```python
from build123d import *

# Parameters (mm, degrees)
SKETCH_1_W          = 26
SKETCH_1_H          = 38
EXTRUDE_1_DEPTH     = 12
SKETCH_2_W          = 22
SKETCH_2_H          = 34
CUT_EXTRUDE_1_DEPTH = 10
SKETCH_3_W          = 2
SKETCH_3_H          = 7
CUT_EXTRUDE_3_DEPTH = 12
SKETCH_4_W          = 6
SKETCH_4_H          = 6
EXTRUDE_2_DEPTH     = 5
SKETCH_5_R          = 1
CUT_EXTRUDE_4_DEPTH = 13
CUT_EXTRUDE_START   = 1
CUT_EXTRUDE_5_DEPTH = 4
SKETCH_7_R          = 12
SKETCH_7_R_2        = 11
EXTRUDE_3_DEPTH     = 5
SKETCH_9_W          = 8
SKETCH_9_H          = 15
CUT_EXTRUDE_7_DEPTH = 1
SKETCH_10_W         = 14.41096837
SKETCH_10_H         = 3
EXTRUDE_4_DEPTH     = 2


with BuildPart() as part:
    # ｽｹｯﾁ1 → ﾎﾞｽ - 押し出し1 (new body)
    with BuildSketch(Plane.XY):
        Rectangle(SKETCH_1_W, SKETCH_1_H)
    extrude(amount=EXTRUDE_1_DEPTH)

    # ｽｹｯﾁ2 → ｶｯﾄ - 押し出し1 (cut)
    with BuildSketch(Plane.XY):
        Rectangle(SKETCH_2_W, SKETCH_2_H)
    extrude(amount=CUT_EXTRUDE_1_DEPTH, mode=Mode.SUBTRACT)

    # ｽｹｯﾁ3 → ｶｯﾄ - 押し出し3 (cut)
    with BuildSketch(Plane.XY):
        with Locations((0.147807357, 5.5)):
            Rectangle(SKETCH_3_W, SKETCH_3_H)
    extrude(amount=CUT_EXTRUDE_3_DEPTH, mode=Mode.SUBTRACT)

    # ｽｹｯﾁ4 → ﾎﾞｽ - 押し出し2 (add)
    with BuildSketch(Plane.XY):
        with Locations((16, 16)):
            Rectangle(SKETCH_4_W, SKETCH_4_H)
        with Locations((16, -16)):
            Rectangle(SKETCH_4_W, SKETCH_4_H)
        with Locations((-16, -16)):
            Rectangle(SKETCH_4_W, SKETCH_4_H)
        with Locations((-16, 16)):
            Rectangle(SKETCH_4_W, SKETCH_4_H)
    extrude(amount=EXTRUDE_2_DEPTH)

    # ｽｹｯﾁ5 → ｶｯﾄ - 押し出し4 (cut, through all)
    with BuildSketch(Plane.XY):
        with Locations((-16, 16)):
            Circle(SKETCH_5_R)
        with Locations((-16, -16)):
            Circle(SKETCH_5_R)
        with Locations((16, -16)):
            Circle(SKETCH_5_R)
        with Locations((16, 16)):
            Circle(SKETCH_5_R)
    extrude(amount=CUT_EXTRUDE_4_DEPTH, mode=Mode.SUBTRACT)

    # ｽｹｯﾁ6 → ｶｯﾄ - 押し出し5 (cut)
    with BuildSketch(Plane.XY.offset(CUT_EXTRUDE_START)):
        Polygon((-17.184124892, 17.98272075), (-18.309148984, 15.965878137), (-17.125024092, 13.983157387), (-14.815875108, 14.01727925), (-13.690851016, 16.034121863), (-14.874975908, 18.016842613), align=None)
        Polygon((-17.07560545, -13.956374239), (-18.307634549, -15.909688764), (-17.2320291, -17.953314524), (-14.92439455, -18.043625761), (-13.692365451, -16.090311236), (-14.7679709, -14.046685476), align=None)
        Polygon((14.939341307, 18.051423035), (13.693086191, 16.107154145), (14.753744884, 14.055731109), (17.060658693, 13.948576965), (18.306913809, 15.892845855), (17.246255116, 17.944268891), align=None)
        Polygon((14.854466591, -13.994735294), (13.690623119, -15.98942868), (14.836156527, -17.994693386), (17.145533409, -18.005264706), (18.309376881, -16.01057132), (17.163843473, -14.005306614), align=None)
    extrude(amount=CUT_EXTRUDE_5_DEPTH, mode=Mode.SUBTRACT)

    # ｽｹｯﾁ7 → ﾎﾞｽ - 押し出し3 (add)
    with BuildSketch(Plane.XY.offset(12)):
        with Locations((0, 5)):
            Circle(SKETCH_7_R)
        with Locations((0, 5)):
            Circle(SKETCH_7_R_2, mode=Mode.SUBTRACT)
    extrude(amount=EXTRUDE_3_DEPTH)

    # ｽｹｯﾁ9 → ｶｯﾄ - 押し出し7 (cut)
    with BuildSketch(Plane.XY.offset(12)):
        with Locations((0.061272904, 4.367214105)):
            Rectangle(SKETCH_9_W, SKETCH_9_H)
    extrude(amount=-CUT_EXTRUDE_7_DEPTH, mode=Mode.SUBTRACT)

    # ｽｹｯﾁ10 → ﾎﾞｽ - 押し出し4 (add)
    with BuildSketch(Plane.XY.offset(10)):
        with Locations((0, -11.5)):
            Rectangle(SKETCH_10_W, SKETCH_10_H)
    extrude(amount=-EXTRUDE_4_DEPTH)


solid = part.part
```
The model under review builds one solid part; all positions refer to its coordinate system, in mm. A direction names the side the tool comes from. Give positions to 0.01 mm unless a question says otherwise; leave off trailing zeros. Write each loop counter-clockwise with the first axis right and the second up, starting at its lowest first coordinate (ties: lowest second). Pieces come first, ordered by that corner, then holes. Notation, with made-up numbers: M 41.25,-29 L 61.25,-29 A15 cw 61.25,0 Z; hole C -30,-36 d7. An arc over 180 degrees is marked long. Write each question's results on one line, items separated by ' | '. Start each with the question number.
1. For probe 1 along Y at (x, z) = (-16, 0.7); probe 2 along X at (y, z) = (16, 0.75); probe 3 along Y at (x, z) = (-2.5, 9.5), list the stretches that pass through material, from the lowest coordinate up. Write a range as [from, to].
2. We need section A-A (z = 9.25). Write out the cut boundary in (x, y), and give its area (3 significant figures).
3. For faces 1 (the flat face through (0.1, 2, 10.5)), 2 (the flat face through (14.255, -16.978, 2.972)), 3 (the flat face through (0, -17, 5)), 4 (the flat face through (18, -15, 5)), 5 (the flat face through (-19, 16, 2)), list the 3-axis set-ups (+Z, -Z, +X, -X, +Y, -Y) from which the entire face can be reached by the end or side of a thin tool; tool diameter is ignored.
4. We need section B-B (x = 0). Write out the cut boundary in (y, z).
5. Insertion check: pin 1 Ø5 at (x, y) = (-16.5, 16) entering from +Z; pin 2 Ø2.5 at (x, y) = (0.5, 3.5) entering from +Z; pin 3 Ø1 at (y, z) = (4.5, 2) entering from +X. Each pin has a flat end and moves straight along its axis. Give the tip position at first contact, or say it passes through.
6. We need section D-D (y = -8.5). Write out the cut boundary in (x, z).
7. We need section C-C (y = 5). Write out the cut boundary in (x, z).
8. Mouldability with a two-part tool opening along Y and no side actions: class faces 6 (the flat face through (4.061, 4.3, 11.5)), 7 (the flat face through (-14.275, 17.012, 2.972)), 8 (the cylindrical face through (-11.99, 5.53, 14.46)), 9 (the flat face through (5, -5, 17)) as released by +Y, released by -Y, zero draft, split by the parting line, or undercut.
Results found:
1) probe 1: y = [-19, -17], [-15, -13], [13, 15], [17, 19] | probe 2: x = [-19, -17], [-15, -11], [11, 15], [17, 19] | probe 3: y = [-19, -17], [-13, -10], [17, 19]
2) outline: M -13,-19 L 13,-19 L 13,19 L -13,19 Z; M -7.21,-13 L 7.21,-13 L 7.21,-10 L -7.21,-10 Z; hole M -11,-17 L 11,-17 L 11,17 L -11,17 Z | area: 283 mm^2
3) face 1: +Z, -Z | face 2: +Z | face 3: -Z | face 4: +Z, +X, +Y, -Y | face 5: +Z, -Z, -X, +Y, -Y
4) outline: M -19,0 L -17,0 L -17,10 L -13,10 L -13,8 L -10,8 L -10,10 L 2,10 L 2,11 L -3.13,11 L -3.13,12 L -6,12 L -6,17 L -7,17 L -7,12 L -19,12 Z; M 9,10 L 17,10 L 17,0 L 19,0 L 19,12 L 17,12 L 17,17 L 16,17 L 16,12 L 11.87,12 L 11.87,11 L 9,11 Z
5) pin 1: stops at z = 5 | pin 2: stops at z = 11 | pin 3: stops at x = 13
6) outline: M -13,0 L -11,0 L -11,10 L 11,10 L 11,0 L 13,0 L 13,12 L -13,12 Z
7) outline: M -13,0 L -11,0 L -11,10 L -0.85,10 L -0.85,11 L -3.94,11 L -3.94,12 L -11,12 L -11,17 L -12,17 L -12,12 L -13,12 Z; M 1.15,10 L 11,10 L 11,0 L 13,0 L 13,12 L 12,12 L 12,17 L 11,17 L 11,12 L 4.06,12 L 4.06,11 L 1.15,11 Z
8) face 6: undercut | face 7: undercut | face 8: split by the parting line | face 9: zero draft
